from build123d import *

# Parameters (mm, degrees)
SKETCH_1_W               = 40
SKETCH_1_H               = 39
CUT_EXTRUDE_1_DEPTH      = 3
CUT_EXTRUDE_2_DEPTH      = 3
CUT_EXTRUDE_3_DEPTH      = 3
CUT_EXTRUDE_4_DEPTH      = 3
CUT_EXTRUDE_5_DEPTH      = 3
CUT_EXTRUDE_6_DEPTH      = 3
HOLE_WIZARD_3_5_3_5_1_D  = 3.5
SKETCH_14_R              = 40
SKETCH_14_R_2            = 37
EXTRUDE_1_DEPTH          = 3
EXTRUDE_2_DEPTH          = 10
FILLET_1_R               = 5
FILLET_2_R               = 5
CUT_EXTRUDE_8_REACH      = 80.109
SKETCH_20_R              = 1.45
CUT_EXTRUDE_9_DEPTH      = 10
CUT_EXTRUDE_9_DEPTH_BACK = 3.1
SKETCH_21_R              = 3.121637526
SKETCH_21_R_2            = 2.750833309
SKETCH_21_R_3            = 2.66


with BuildPart() as part:
    # 草图1 → 旋转1 (revolve)
    with BuildSketch(Plane.XY, mode=Mode.PRIVATE) as revolve_1_sk:
        with Locations((20, 19.5)):
            Rectangle(SKETCH_1_W, SKETCH_1_H)
    revolve(revolve_1_sk.sketch.rotate(Axis((0, 39, 0), (0, -1, 0)), 270), axis=Axis((0, 39, 0), (0, -1, 0)))

    # 草图2 → M64 六角头螺栓的柱形沉头孔1 (revolve, cut)
    with BuildSketch(Plane(origin=(0, 39, 0), x_dir=(0, 0, 1), z_dir=(1, 0, 0))):
        Polygon((0, 0), (0, 39), (37, 39), (37, 5), (21.5, 5), (21.5, 0), align=None)
    revolve(axis=Axis((0, 45.35, 0), (0, -1, 0)), mode=Mode.SUBTRACT)

    # 草图4 → 切除-拉伸1 (cut)
    with BuildSketch(Plane.XZ.offset(-34)):
        Polygon((16.100028232, 27.856820067), (15.750000921, 24.52653266), (18.459100762, 22.558256413), (21.518227914, 23.920267573), (21.868255226, 27.25055498), (19.159155385, 29.218831227), align=None)
    extrude(amount=-CUT_EXTRUDE_1_DEPTH, mode=Mode.SUBTRACT)

    # 草图5 → 切除-拉伸2 (cut)
    with BuildSketch(Plane.XZ.offset(-34)):
        Polygon((-21.868255226, 27.25055498), (-21.518227914, 23.920267573), (-18.459100762, 22.558256413), (-15.750000921, 24.52653266), (-16.100028232, 27.856820067), (-19.159155385, 29.218831227), align=None)
    extrude(amount=-CUT_EXTRUDE_2_DEPTH, mode=Mode.SUBTRACT)

    # 草图6 → 切除-拉伸3 (cut)
    with BuildSketch(Plane.XZ.offset(-34)):
        Polygon((-18.459100762, -22.558256413), (-21.518227914, -23.920267573), (-21.868255226, -27.25055498), (-19.159155385, -29.218831227), (-16.100028232, -27.856820067), (-15.750000921, -24.52653266), align=None)
    extrude(amount=-CUT_EXTRUDE_3_DEPTH, mode=Mode.SUBTRACT)

    # 草图7 → 切除-拉伸4 (cut)
    with BuildSketch(Plane.XZ.offset(-34)):
        Polygon((1.674315781, -29.1), (-1.674315781, -29.1), (-3.348631561, -32), (-1.674315781, -34.9), (1.674315781, -34.9), (3.348631561, -32), align=None)
    extrude(amount=-CUT_EXTRUDE_4_DEPTH, mode=Mode.SUBTRACT)

    # 草图8 → 切除-拉伸5 (cut)
    with BuildSketch(Plane.XZ.offset(-34)):
        Polygon((21.868255226, -27.25055498), (21.518227914, -23.920267573), (18.459100762, -22.558256413), (15.750000921, -24.52653266), (16.100028232, -27.856820067), (19.159155385, -29.218831227), align=None)
    extrude(amount=-CUT_EXTRUDE_5_DEPTH, mode=Mode.SUBTRACT)

    # 草图9 → 切除-拉伸6 (cut)
    with BuildSketch(Plane.XZ.offset(-34)):
        Polygon((-3.348631561, 32), (-1.674315781, 29.1), (1.674315781, 29.1), (3.348631561, 32), (1.674315781, 34.9), (-1.674315781, 34.9), align=None)
    extrude(amount=-CUT_EXTRUDE_6_DEPTH, mode=Mode.SUBTRACT)

    # Ø3.5 (3.5) 直径孔1 (through all)
    with Locations(Plane(origin=(0, 37, 0), x_dir=(-1, 0, 0), z_dir=(0, -1, 0))):
        with Locations((18.809128073, 25.88854382), (-18.809128073, 25.88854382), (0, 32), (18.809128073, -25.88854382), (-18.809128073, -25.88854382), (0, -32)):
            Hole(HOLE_WIZARD_3_5_3_5_1_D / 2)

    # 草图14 → 凸台-拉伸1 (add)
    with BuildSketch(Plane.XZ):
        with Locations(Location((0, 0, 0), (0, 0, 270))):
            Circle(SKETCH_14_R)
        with Locations(Location((0, 0, 0), (0, 0, 90))):
            Circle(SKETCH_14_R_2, mode=Mode.SUBTRACT)
    extrude(amount=EXTRUDE_1_DEPTH)

    # 草图15 → 凸台-拉伸2 (add)
    with BuildSketch(Plane.XZ.offset(3)):
        Polygon((29.327322558, 27.208971895), (38.222658937, 11.791028105), (43.998438168, 21.790578059), (40.875075675, 27.204181918), align=None)
        Polygon((8.899999593, -39.002692308), (-8.899999593, -38.997307692), (-3.128024922, -48.99905421), (3.121974792, -49.000944875), align=None)
        Polygon((-38.227322151, 11.793720413), (-29.322659344, 27.206279587), (-40.870413246, 27.208476151), (-43.997050467, 21.796762958), align=None)
    extrude(amount=-EXTRUDE_2_DEPTH)

    # 圆角1
    # the kernel refuses this fillet: 5 mm, written as the material it adds along each edge
    with BuildSketch(Plane(origin=(0, 7, 0), x_dir=(0, 0, -1), z_dir=(1, 0, 0))) as fillet_1_piece_1_section:
        with BuildLine():
            CenterArc((40 + FILLET_1_R, FILLET_1_R), FILLET_1_R, 180, 90)
            Line((40 + FILLET_1_R, 0), (40, 0))
            Line((40, 0), (40, FILLET_1_R))
        make_face()
    fillet_1_piece_1 = revolve(axis=Axis((0, 7, 0), (0, 1, 0)), revolution_arc=30.760989805, mode=Mode.PRIVATE)
    fillet_1_piece_1 = split(fillet_1_piece_1, bisect_by=Plane(origin=(-6.938848229, 8.159603728, -42.395614154), z_dir=(0.866120495946599, 0, 0.4998352593617396)), keep=Keep.TOP, mode=Mode.PRIVATE)
    add(fillet_1_piece_1)
    with BuildSketch(Plane(origin=(0, 7, 0), x_dir=(0.510937919824611, 0, -0.8596176138756695), z_dir=(0.8596176138756695, 0, 0.510937919824611))) as fillet_1_piece_2_section:
        with BuildLine():
            CenterArc((40 + FILLET_1_R, FILLET_1_R), FILLET_1_R, 180, 90)
            Line((40 + FILLET_1_R, 0), (40, 0))
            Line((40, 0), (40, FILLET_1_R))
        make_face()
    fillet_1_piece_2 = revolve(axis=Axis((0, 7, 0), (0, 1, 0)), revolution_arc=30.726324325, mode=Mode.PRIVATE)
    fillet_1_piece_2 = split(fillet_1_piece_2, bisect_by=Plane(origin=(4.116270695, 8.159650312, -39.001245199), z_dir=(-0.0003025064822812723, 0, -0.9999999542449131)), keep=Keep.TOP, mode=Mode.PRIVATE)
    fillet_1_piece_2 = split(fillet_1_piece_2, bisect_by=Plane(origin=(6.938556974, 8.159650312, -42.396758511), z_dir=(-0.865817930630708, 0, 0.500359181986659)), keep=Keep.TOP, mode=Mode.PRIVATE)
    add(fillet_1_piece_2)

    # 圆角2
    # the kernel refuses this fillet: 5 mm, written as the material it adds along each edge
    with BuildSketch(Plane(origin=(0, 7, 0), x_dir=(-0.9999195538304662, 0, -0.01268407929183255), z_dir=(0.01268407929183255, 0, -0.9999195538304662))) as fillet_2_piece_1_section:
        with BuildLine():
            CenterArc((40 + FILLET_2_R, FILLET_2_R), FILLET_2_R, 180, 90)
            Line((40, FILLET_2_R), (40, 0))
            Line((40, 0), (40 + FILLET_2_R, 0))
        make_face()
    fillet_2_piece_1 = revolve(axis=Axis((0, 7, 0), (0, 1, 0)), revolution_arc=61.488192088, mode=Mode.PRIVATE)
    fillet_2_piece_1 = split(fillet_2_piece_1, bisect_by=Plane(origin=(-33.775857592, 8.159626542, 19.49849963), z_dir=(-0.8658741109182307, 0, 0.5002619554209213)), keep=Keep.TOP, mode=Mode.PRIVATE)
    fillet_2_piece_1 = split(fillet_2_piece_1, bisect_by=Plane(origin=(-41.214638413, 8.159626542, 16.972864045), z_dir=(0.8662327279326016, 0, 0.4996407319849368)), keep=Keep.TOP, mode=Mode.PRIVATE)
    fillet_2_piece_1 = split(fillet_2_piece_1, bisect_by=Plane(origin=(-35.303320955, 8.159626542, 27.207417203), z_dir=(-0.00019021565884901444, 0, -0.9999999819090014)), keep=Keep.TOP, mode=Mode.PRIVATE)
    add(fillet_2_piece_1)
    with BuildSketch(Plane(origin=(0, 7, 0), x_dir=(0.4889750420250284, 0, 0.8722977750038238), z_dir=(-0.8722977750038238, 0, 0.4889750420250284))) as fillet_2_piece_2_section:
        with BuildLine():
            CenterArc((40 + FILLET_2_R, FILLET_2_R), FILLET_2_R, 180, 90)
            Line((40, FILLET_2_R), (40, 0))
            Line((40, 0), (40 + FILLET_2_R, 0))
        make_face()
    fillet_2_piece_2 = revolve(axis=Axis((0, 7, 0), (0, 1, 0)), revolution_arc=61.488192088, mode=Mode.PRIVATE)
    fillet_2_piece_2 = split(fillet_2_piece_2, bisect_by=Plane(origin=(33.774124811, 8.159626542, 19.501500894), z_dir=(0.8661766174005117, 0, 0.49973799882399134)), keep=Keep.TOP, mode=Mode.PRIVATE)
    fillet_2_piece_2 = split(fillet_2_piece_2, bisect_by=Plane(origin=(35.306250644, 8.159626542, 27.206491851), z_dir=(-0.0004147973018910844, 0, -0.9999999139715955)), keep=Keep.TOP, mode=Mode.PRIVATE)
    fillet_2_piece_2 = split(fillet_2_piece_2, bisect_by=Plane(origin=(41.213974946, 8.159626542, 16.969864183), z_dir=(-0.8659302802877497, 0, 0.5001647225472617)), keep=Keep.TOP, mode=Mode.PRIVATE)
    add(fillet_2_piece_2)

    # 草图20 → 切除-拉伸8 (cut, up to next)
    with BuildSketch(Plane.XZ.offset(3), mode=Mode.PRIVATE) as cut_extrude_8_sk1:
        with Locations(Location((0.000280142, -44.000000314, 0), (0, 0, 270))):
            Circle(SKETCH_20_R)
    cut_extrude_8_tool1 = extrude(cut_extrude_8_sk1.sketch, amount=-CUT_EXTRUDE_8_REACH, mode=Mode.PRIVATE) & part.part
    # 草图20 → 切除-拉伸8 (cut, up to next)
    with BuildSketch(Plane.XZ.offset(3), mode=Mode.PRIVATE) as cut_extrude_8_sk2:
        with Locations(Location((-38.105258109, 21.999757547, 0), (0, 0, 270))):
            Circle(SKETCH_20_R)
    cut_extrude_8_tool2 = extrude(cut_extrude_8_sk2.sketch, amount=-CUT_EXTRUDE_8_REACH, mode=Mode.PRIVATE) & part.part
    # 草图20 → 切除-拉伸8 (cut, up to next)
    with BuildSketch(Plane.XZ.offset(3), mode=Mode.PRIVATE) as cut_extrude_8_sk3:
        with Locations(Location((38.104977967, 22.000242767, 0), (0, 0, 270))):
            Circle(SKETCH_20_R)
    cut_extrude_8_tool3 = extrude(cut_extrude_8_sk3.sketch, amount=-CUT_EXTRUDE_8_REACH, mode=Mode.PRIVATE) & part.part
    add(cut_extrude_8_tool1.solids().sort_by_distance((0.00028, -3, -44))[0], mode=Mode.SUBTRACT)
    add(cut_extrude_8_tool2.solids().sort_by_distance((-38.105258, -3, 21.999758))[0], mode=Mode.SUBTRACT)
    add(cut_extrude_8_tool3.solids().sort_by_distance((38.104978, -3, 22.000243))[0], mode=Mode.SUBTRACT)

    # 草图21 → 切除-拉伸9 (cut, two sides: drawn at the far end of the back side and taken through both)
    # profile 1 of 4: a face of its own
    with BuildSketch(Plane(origin=(0, 7, 0), x_dir=(1, 0, 0), z_dir=(0, 1, 0)).offset(-CUT_EXTRUDE_9_DEPTH_BACK)):
        Circle(SKETCH_21_R)
        Circle(SKETCH_21_R_2, mode=Mode.SUBTRACT)
    # profile 2 of 4: a face of its own
    with BuildSketch(Plane(origin=(0, 7, 0), x_dir=(1, 0, 0), z_dir=(0, 1, 0)).offset(-CUT_EXTRUDE_9_DEPTH_BACK)):
        with Locations(Location((0.000280142, 44.000000314, 0), (0, 0, 159.513268141))):
            Circle(SKETCH_21_R_3)
    # profile 3 of 4: a face of its own
    with BuildSketch(Plane(origin=(0, 7, 0), x_dir=(1, 0, 0), z_dir=(0, 1, 0)).offset(-CUT_EXTRUDE_9_DEPTH_BACK)):
        with Locations(Location((38.104977967, -22.000242767, 0), (0, 0, 39.513268136))):
            Circle(SKETCH_21_R_3)
    # profile 4 of 4: a face of its own
    with BuildSketch(Plane(origin=(0, 7, 0), x_dir=(1, 0, 0), z_dir=(0, 1, 0)).offset(-CUT_EXTRUDE_9_DEPTH_BACK)):
        with Locations(Location((-38.105258109, -21.999757547, 0), (0, 0, 140.486002271))):
            Circle(SKETCH_21_R_3)
    extrude(amount=CUT_EXTRUDE_9_DEPTH + CUT_EXTRUDE_9_DEPTH_BACK, mode=Mode.SUBTRACT)


solid = part.part
Input: part model. Units: mm. Frame: model coordinates. A direction names the side the tool comes from. Round coordinates to 2 decimals unless told otherwise and drop trailing zeros. Write each loop counter-clockwise with the first axis right and the second up, starting at its lowest first coordinate (ties: lowest second). Pieces come first, ordered by that corner, then holes.
1) Cut plane A-A (z = 7). Return the cut outline in (x, y), then the cut area to 3 significant figures.
2) Contact query for flat-ended pins moving along their axis: P1, Ø5.5, axis at x = -31, y = 9.5, coming from the +Z side; P2, Ø5, axis at x = 0, z = -44, coming from the -Y side; P3, Ø1, axis at x = 6, y = 28, coming from the -Z side; P4, Ø2.5, axis at x = -38, z = 22.5, coming from the +Y side. Output: stop coordinate, or through.
3) Cut plane C-C (y = 18). Return the cut outline in (x, z), then the cut area to 3 significant figures.
4) Ray query, L1, parallel to Y at x = 5, z = -34; L2, parallel to Z at x = -9.5, y = 33.5; L3, parallel to X at y = 27.5, z = 0.5. Return the intervals inside material, ascending.
5) Reachability of faces 1 (the flat face through (1.4, 37, 33.3)), 2 (the cylindrical face through (18.581, 38.014, 24.153)), 3 (the flat face through (-0.7, 3.9, -45.5)) from +Z, -Z, +X, -X, +Y, -Y: full face, straight path, thin tool, end or side. Return the list, or none.
6) Draft query along X for faces 4 (the flat face through (-17, 39, 17)), 5 (the cylindrical face through (-20.1, 38.01, -27.07)), 6 (the cylindrical face through (-39.05, 18.29, 8.67)). Return one class per face: pulls with the +X half, pulls with the -X half, needs draft (parallel to the pull), parting line crosses it, or undercut.
Geometry says:
1. outline: (-39.38, -3) - (-36.33, -3) - (-36.33, 34) - (-20.33, 34) - (-20.33, 39) - (-39.38, 39) - close; (20.33, 34) - (36.33, 34) - (36.33, -3) - (39.38, -3) - (39.38, 39) - (20.33, 39) - close
1. area: 416 mm2
2. P1: stops at z = 28.32
2. P2: stops at y = -3
2. P3: stops at z = -39.62
2. P4: stops at y = 3.9
3. outline: circle Ø80 at (0, 0); hole circle Ø74 at (0, 0)
3. area: 726 mm2
4. L1: y = 34 to 39
4. L2: z = -38.86 to -35.76, 35.76 to 38.86
4. L3: x = -40 to -37, 37 to 40
5. face 1: -Y
5. face 2: +Y, -Y
5. face 3: +Y
6. face 4: needs draft
6. face 5: undercut
6. face 6: parting line crosses it
